Design review of the part built by this model. Coordinates are the model's own, in mm. Face numbers are marked on the shaded views. Coordinates: 2 decimals unless noted, no trailing zeros. Order: outer loops, then holes, each group sorted by start corner. A loop starts at its lowest first (then second) coordinate and runs counter-clockwise, first axis right, second up. Notation, with made-up numbers: (-17, 87.5) - (34, 87.5) arc R9 ccw to (34, 94.5) - close; hole circle Ø5 at (47, -3.5). An arc over 180 degrees is marked (long way). Write each question's results on one line, items separated by ' | '. Start each with the question number.
```python
from build123d import *

# Parameters (mm, degrees)
F0_W      = 20
F0_H      = 50
F0_H_2    = 2
F1_DEPTH  = 8
F3_DEPTH  = 50
F4_DEPTH  = 25.4
F5_T      = -2
F6_W      = 2
F6_H      = 5
F6_H_2    = 2
F6_W_2    = 20
F6_W_3    = 43.6544959545
F6_H_3    = 1
F6_H_4    = 3
F7_DEPTH  = 8
F9_DEPTH  = 76.2
F10_DEPTH = 6


with BuildPart() as f1:
    # F0 (on Front) → F1 (new body)
    with BuildSketch(Plane.XZ):
        Polygon((12, 27), (-12, 27), (-12, -27), (-10, -27), (-10, -25), (-10, 25), (10, 25), (10, -25), (10, -27), (12, -27), align=None)
        Rectangle(F0_W, F0_H)
        with Locations((0, -26)):
            Rectangle(F0_W, F0_H_2)
    extrude(amount=F1_DEPTH)

    # F2 (on Right) → F3 (cut)
    with BuildSketch(Plane.YZ):
        Polygon((-6.5, 23.2472232503), (-1.5, 26.1339745962), (0, 27), (-8, 27), (-8, 22.3811978465), align=None)
    extrude(amount=-F3_DEPTH, mode=Mode.SUBTRACT)

    # F2 (on Right) → F4 (cut)
    with BuildSketch(Plane.YZ):
        Polygon((-6.5, 23.2472232503), (-1.5, 26.1339745962), (0, 27), (-8, 27), (-8, 22.3811978465), align=None)
    extrude(amount=F4_DEPTH, mode=Mode.SUBTRACT)

    # F5
    f5_openings = [f1.faces().sort_by_distance(p)[0] for p in [
        (0, 0, 0),
        (0, -4, -27),
    ]]
    offset(amount=F5_T, openings=f5_openings)

    # F6 (on face) → F7 (join)
    with BuildSketch(Plane(origin=(0, 0, 0), x_dir=(-1, 0, 0), z_dir=(0, 1, 0))):
        with Locations((11, -29.5)):
            Rectangle(F6_W, F6_H)
        with Locations((11, -33)):
            Rectangle(F6_W, F6_H_2)
        with Locations((0, -33)):
            Rectangle(F6_W_2, F6_H_2)
        with Locations((-31.8272479773, -33)):
            Rectangle(F6_W_3, F6_H_2)
        Polygon((-10, -28), (-10, -27), (-12, -27), (-53.6544959545, -27), (-53.6544959545, -28), align=None)
        with Locations((-54.6544959545, -27.5)):
            Rectangle(F6_W, F6_H_3)
        with Locations((-54.6544959545, -30.5)):
            Rectangle(F6_W, F6_H_4)
        with Locations((-54.6544959545, -33)):
            Rectangle(F6_W, F6_H_2)
        Polygon((10, -32), (10, -27), (-10, -27), (-10, -28), (-10, -29), (-53.6544959545, -29), (-53.6544959545, -32), (-10, -32), align=None)
        with Locations((-31.8272479773, -28.5)):
            Rectangle(F6_W_3, F6_H_3)
        with Locations((-54.6544959545, -28.5)):
            Rectangle(F6_W, F6_H_3)
    extrude(amount=-F7_DEPTH)

    # F8 (on face) → F9 (cut)
    with BuildSketch(Plane.YZ.offset(55.6544959545)):
        Polygon((-1, -27), (-8, -34), (0, -34), (0, -27), align=None)
    extrude(amount=-F9_DEPTH, mode=Mode.SUBTRACT)

    # F6 (on face) → F10 (cut)
    with BuildSketch(Plane(origin=(0, 0, 0), x_dir=(-1, 0, 0), z_dir=(0, 1, 0))):
        Polygon((10, -32), (10, -27), (-10, -27), (-10, -28), (-10, -29), (-53.6544959545, -29), (-53.6544959545, -32), (-10, -32), align=None)
    extrude(amount=-F10_DEPTH, mode=Mode.SUBTRACT)


solid = f1.part
```
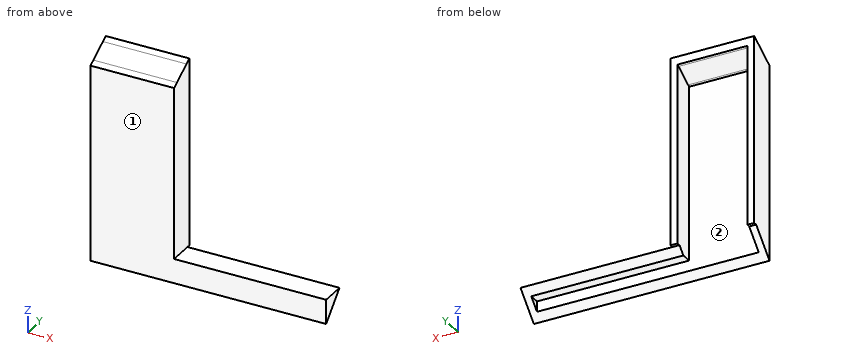
(1) Mouldability with a two-part tool opening along X and no side actions: class the marked faces 1 and 2 as +X half, -X half, draft (parallel to the pull), parting line (faces both ways), or undercut.
(2) Take a section at B-B (z = -28). State the section outline as (x, y) points.
(3) Take a section at A-A (x = 14). State the section outline as (y, z) points.
(4) Take a section at C-C (y = -4.5). State the section outline as (x, z) points, plus the area to 3 significant figures.
(5) Take a section at D-D (z = -8). State the section outline as (x, y) points, plus the area to 3 significant figures.
(6) Clearance check with flat-ended pins moving along their axes: pin 1 (2.5 mm diameter, centred on y = -4.5, z = -2, fed in from +X); pin 2 (2.5 mm diameter, centred on x = 23.5, y = -5, fed in from -Z). State where each tip first meets the part, or that it passes through.
(7) To check wall thickness, follow line 1 along X through (y, z) = (-5, -13.5); line 2 along Y through (x, z) = (-2.5, -7); line 3 along Z through (x, y) = (25, -3.5). State the ranges of each line that lie inside material, in increasing order. Write a range as [from, to].
Worked out:
1) face 1: draft | face 2: undercut
2) outline: (-12, -8) - (55.65, -8) - (55.65, -2) - (10, -2) - (10, -6) - (-10, -6) - (-10, -2) - (-12, -2) - close
3) outline: (-8, -34) - (-6, -32) - (-6, -29) - (-3, -29) - (-1, -27) - (-8, -27) - close
4) outline: (-12, -30.5) - (-10, -30.5) - (-10, 22.09) - (10, 22.09) - (10, -29) - (53.65, -29) - (53.65, -30.5) - (55.65, -30.5) - (55.65, -27) - (12, -27) - (12, 24.4) - (-12, 24.4) - close | area: 353 mm^2
5) outline: (-12, -8) - (12, -8) - (12, 0) - (10, 0) - (10, -6) - (-10, -6) - (-10, 0) - (-12, 0) - close | area: 72.0 mm^2
6) pin 1: x = 12 | pin 2: z = -32.25
7) line 1: [-12, -10], [10, 12] | line 2: [-8, -6] | line 3: [-29, -27]
